Geometry check sheet. Reference: the model listing, model coordinates, mm. A direction names the side the tool comes from. Give positions to 0.01 mm unless a question says otherwise; leave off trailing zeros. Write each loop counter-clockwise with the first axis right and the second up, starting at its lowest first coordinate (ties: lowest second). Pieces come first, ordered by that corner, then holes. Notation, with made-up numbers: (-31.5, 79) -> (24.5, 79) arc R8 ccw to (24.5, 86) -> close; hole circle Ø7 at (-6, 49). An arc over 180 degrees is marked (long way). One line per item, written item: value.
from build123d import *

# Parameters (mm, degrees)
SKETCH7_W          = 12
SKETCH7_H          = 4
CUT_EXTRUDE4_DEPTH = 3.2


with BuildPart() as part:
    # Sketch6 → Revolve2 (revolve)
    with BuildSketch(Plane.XY, mode=Mode.PRIVATE) as revolve2_sk:
        Polygon((-52.75, 4.5), (-52.75, 7), (-42.75, 7), (-42.75, 10), (-35.75, 10), (-35.75, 12), (-28.25, 12), (-28.25, 11), (44.75, 11), (44.75, 8.5), (52.75, 8.5), (52.75, 4.5), align=None)
    revolve(revolve2_sk.sketch.rotate(Axis((-52.75, 0, 0), (1, 0, 0)), 180), axis=Axis((-52.75, 0, 0), (1, 0, 0)))

    # Sketch7 → Cut-Extrude4 (cut)
    with BuildSketch(Plane(origin=(0, 11, 0), x_dir=(1, 0, 0), z_dir=(0, 1, 0))):
        with Locations((8.25, 0)):
            Rectangle(SKETCH7_W, SKETCH7_H)
    extrude(amount=-CUT_EXTRUDE4_DEPTH, mode=Mode.SUBTRACT)


solid = part.part
1) Sectioned sample at B-B on y = 0. Record the cut outline in (x, z), plus the area to 3 significant figures.
Verdict:
outline: (-52.75, -7) -> (-42.75, -7) -> (-42.75, -10) -> (-35.75, -10) -> (-35.75, -12) -> (-28.25, -12) -> (-28.25, -11) -> (44.75, -11) -> (44.75, -8.5) -> (52.75, -8.5) -> (52.75, -4.5) -> (-52.75, -4.5) -> close; (-52.75, 4.5) -> (52.75, 4.5) -> (52.75, 8.5) -> (44.75, 8.5) -> (44.75, 11) -> (-28.25, 11) -> (-28.25, 12) -> (-35.75, 12) -> (-35.75, 10) -> (-42.75, 10) -> (-42.75, 7) -> (-52.75, 7) -> close
area: 1,250 mm^2
2) Depth check by flat-ended pin: pin 1 Ø2.5 at (y, z) = (8.5, 0) entering from -X; pin 2 Ø8 at (x, y) = (-4.5, -9) entering from +Z; pin 3 Ø2 at (x, z) = (10, -0.5) entering from +Y. Enter the tip coordinate at first touch or a pass-through.
Verdict:
pin 1: x = -42.75
pin 2: z = 9.8
pin 3: y = 7.8
3) Tool access check on faces 1 (the cylindrical face through (8.761, -10.161, 4.213)), 2 (the cylindrical face through (-31.947, -11.446, -3.604)), 3 (the flat face through (-35.75, -5, -9)), 4 (the flat face through (8, 9, -2)). Record the directions out of +Z, -Z, +X, -X, +Y, -Y that give a thin tool (end or side, any length) a straight path to the whole face; none if there is none.
Verdict:
face 1: +X
face 2: +X, -X
face 3: -X
face 4: +Y
4) Sectioned sample at C-C on x = 7. Record the cut outline in (y, z).
Verdict:
outline: (7.8, -2) -> (7.8, 2) -> (10.82, 2) arc R11 ccw (long way) to (10.82, -2) -> close; hole circle Ø9 at (0, 0)
5) Sectioned sample at D-D on z = -5.5. Record the cut outline in (x, y), plus the area to 3 significant figures.
Verdict:
outline: (-52.75, -4.33) -> (-42.75, -4.33) -> (-42.75, -8.35) -> (-35.75, -8.35) -> (-35.75, -10.67) -> (-28.25, -10.67) -> (-28.25, -9.53) -> (44.75, -9.53) -> (44.75, -6.48) -> (52.75, -6.48) -> (52.75, 6.48) -> (44.75, 6.48) -> (44.75, 9.53) -> (-28.25, 9.53) -> (-28.25, 10.67) -> (-35.75, 10.67) -> (-35.75, 8.35) -> (-42.75, 8.35) -> (-42.75, 4.33) -> (-52.75, 4.33) -> close
area: 1,860 mm^2
6) Mould release check, pull along X, two halves, no side actions. Record for faces 5 (the flat face through (-52.75, 0, 5)), 6 (the flat face through (-28.25, -5, 10)), 7 (the flat face through (8, 7.8, 0)), 8 (the flat face through (14.25, 9, 0)): released by +X, released by -X, zero draft, split by the parting line, or undercut.
Verdict:
face 5: released by -X
face 6: released by +X
face 7: undercut
face 8: undercut
7) Scan lines: probe 1 along Z at (x, y) = (5, 0); probe 2 along X at (y, z) = (10.75, 5); probe 3 along X at (y, z) = (-4.75, 7.5). Record each from-to range of solid material in increasing order.
Verdict:
probe 1: -11 to -4.5, 4.5 to 11
probe 2: -35.75 to -28.25
probe 3: -42.75 to 44.75
8) Sectioned sample at A-A on z = 0. Record the cut outline in (x, y), plus the area to 3 significant figures.
Verdict:
outline: (-52.75, -7) -> (-42.75, -7) -> (-42.75, -10) -> (-35.75, -10) -> (-35.75, -12) -> (-28.25, -12) -> (-28.25, -11) -> (44.75, -11) -> (44.75, -8.5) -> (52.75, -8.5) -> (52.75, -4.5) -> (-52.75, -4.5) -> close; (-52.75, 4.5) -> (52.75, 4.5) -> (52.75, 8.5) -> (44.75, 8.5) -> (44.75, 11) -> (14.25, 11) -> (14.25, 7.8) -> (2.25, 7.8) -> (2.25, 11) -> (-28.25, 11) -> (-28.25, 12) -> (-35.75, 12) -> (-35.75, 10) -> (-42.75, 10) -> (-42.75, 7) -> (-52.75, 7) -> close
area: 1,210 mm^2
